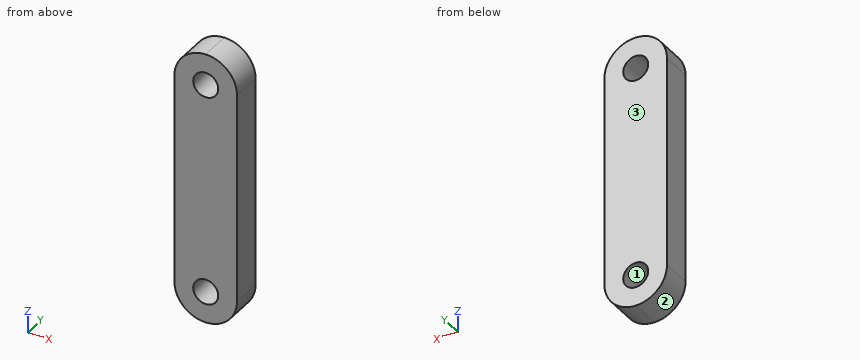
```python
from build123d import *

# Parameters (mm, degrees)
SKETCH1_W           = 8
SKETCH1_H           = 4
BOSS_EXTRUDE1_DEPTH = 35
SKETCH2_R           = 1.6
CUT_EXTRUDE1_DEPTH  = 37.124783736
FILLET1_R           = 4


with BuildPart() as part:
    # Sketch1 → Boss-Extrude1 (new body)
    with BuildSketch(Plane.XY):
        with Locations((4, -2)):
            Rectangle(SKETCH1_W, SKETCH1_H)
    extrude(amount=BOSS_EXTRUDE1_DEPTH)

    # Sketch2 → Cut-Extrude1 (cut, through all)
    with BuildSketch(Plane(origin=(0, 0, 0), x_dir=(1, 0, 0), z_dir=(0, 1, 0))):
        with Locations(Location((4, -4, 0), (0, 0, 270))):
            Circle(SKETCH2_R)
        with Locations(Location((4, -31, 0), (0, 0, 270))):
            Circle(SKETCH2_R)
    extrude(amount=-CUT_EXTRUDE1_DEPTH, mode=Mode.SUBTRACT)

    # Fillet1
    fillet1_edges = [part.edges().sort_by_distance(p)[0] for p in [
        (0, -2, 0),
        (8, -2, 0),
        (0, -2, 35),
        (8, -2, 35),
    ]]
    fillet(fillet1_edges, radius=FILLET1_R - 0.0001)  # a hair under: the kernel refuses the full size


solid = part.part
```
Geometry: final body of the model. Coordinates: model frame, mm. Face numbers are marked on the shaded views. Coordinates: 2 decimals unless noted, no trailing zeros. Order: outer loops, then holes, each group sorted by start corner. A loop starts at its lowest first (then second) coordinate and runs counter-clockwise, first axis right, second up. Notation, with made-up numbers: (69.25, -14.5) - (103.25, -14.5) arc R23 cw to (103.25, -2.5) - close; hole circle Ø8 at (-19.5, 26). An arc over 180 degrees is marked (long way). Write each question's results on one line, items separated by ' | '.
1) Pull-direction query (Z, two-part tool) for the marked faces 1, 2 and 3; classes: pulls with the +Z half, pulls with the -Z half, needs draft (parallel to the pull), parting line crosses it, or undercut.
Results list:
face 1: undercut | face 2: pulls with the -Z half | face 3: needs draft
2) Line query: line 1 (X direction, y = -2, z = 31); line 2 (Z direction, x = 4.5, y = -2.5); line 3 (Z direction, x = 5, y = -2). Output: solid intervals per line, ascending. Write a range as from..to.
Results list:
line 1: 0..2.4, 5.6..8 | line 2: 0.03..2.48, 5.52..29.48, 32.52..34.97 | line 3: 0.13..2.75, 5.25..29.75, 32.25..34.87
3) Section A-A, the plane y = -3.4. State how many separate pieces and enclosed holes the cut face has, plus the area to 3 significant figures.
Results list:
separate pieces: 1 | enclosed holes: 2 | area: 250 mm^2
4) Section B-B, the plane x = 6.5. Return loops of the section in (y, z), plus the area to 3 significant figures.
Results list:
outline: (-4, 0.88) - (0, 0.88) - (0, 34.12) - (-4, 34.12) - close | area: 133 mm^2
